Work out the finished part from the listing and answer in its coordinate system (mm). A direction names the side the tool comes from. Coordinates: 2 decimals unless noted, no trailing zeros. Order: outer loops, then holes, each group sorted by start corner. A loop starts at its lowest first (then second) coordinate and runs counter-clockwise, first axis right, second up.
```python
from build123d import *

# Parameters (mm, degrees)
F0_W      = 15
F0_H      = 15
F1_DEPTH  = 50
F2_W      = 15
F2_H      = 55
F3_DEPTH  = 20
F4_R      = 2.75
F5_DEPTH  = 50.001
F6_R      = 5
F7_DEPTH  = 45
F9_DEPTH  = 2.5
F10_R     = 1.5
F11_DEPTH = 12.501
F13_DEPTH = 2.5
F14_R     = 1.5
F15_DEPTH = 25
F16_R     = 5


with BuildPart() as f1:
    # F0 (on Front) → F1 (new body)
    with BuildSketch(Plane.XZ):
        with Locations((0, 20)):
            Rectangle(F0_W, F0_H)
        with Locations((0, -20)):
            Rectangle(F0_W, F0_H)
    extrude(amount=F1_DEPTH)

    # F2 (on face) → F3 (join)
    with BuildSketch(Plane.XZ.offset(50)):
        Rectangle(F2_W, F2_H)
    extrude(amount=-F3_DEPTH)

    # F4 (on face) → F5 (cut, through all)
    with BuildSketch(Plane(origin=(0, 0, 0), x_dir=(-1, 0, 0), z_dir=(0, 1, 0))):
        with Locations((0, 20)):
            Circle(F4_R)
        with Locations((0, -20)):
            Circle(F4_R)
    extrude(amount=-F5_DEPTH, mode=Mode.SUBTRACT)

    # F6 (on face) → F7 (cut)
    with BuildSketch(Plane.XZ.offset(50)):
        with Locations((0, 20)):
            Circle(F6_R)
        with Locations((0, -20)):
            Circle(F6_R)
    extrude(amount=-F7_DEPTH, mode=Mode.SUBTRACT)

    # F8 (on face) → F9 (cut)
    with BuildSketch(Plane(origin=(-7.5, 0, 0), x_dir=(0, -1, 0), z_dir=(-1, 0, 0))):
        Polygon((35.5, -3.175426), (38.25, -1.587713), (38.25, 1.587713), (35.5, 3.175426), (32.75, 1.587713), (32.75, -1.587713), align=None)
        Polygon((47.25, 1.587713), (44.5, 3.175426), (41.75, 1.587713), (41.75, -1.587713), (44.5, -3.175426), (47.25, -1.587713), align=None)
    extrude(amount=-F9_DEPTH, mode=Mode.SUBTRACT)

    # F10 (on face) → F11 (cut, through all)
    with BuildSketch(Plane(origin=(-5, 0, 0), x_dir=(0, -1, 0), z_dir=(-1, 0, 0))):
        with Locations((35.5, 0)):
            Circle(F10_R)
        with Locations((44.5, 0)):
            Circle(F10_R)
    extrude(amount=-F11_DEPTH, mode=Mode.SUBTRACT)

    # F12 (on face) → F13 (cut)
    with BuildSketch(Plane.XZ.offset(50)):
        Polygon((1.587713, 2), (3.175426, 4.75), (1.587713, 7.5), (-1.587713, 7.5), (-3.175426, 4.75), (-1.587713, 2), align=None)
        Polygon((1.587713, -7.5), (3.175426, -4.75), (1.587713, -2), (-1.587713, -2), (-3.175426, -4.75), (-1.587713, -7.5), align=None)
    extrude(amount=-F13_DEPTH, mode=Mode.SUBTRACT)

    # F14 (on face) → F15 (cut)
    with BuildSketch(Plane.XZ.offset(47.5)):
        with Locations((0, 4.75)):
            Circle(F14_R)
        with Locations((0, -4.75)):
            Circle(F14_R)
    extrude(amount=-F15_DEPTH, mode=Mode.SUBTRACT)

    # F16
    f16_edges = [f1.edges().sort_by_distance(p)[0] for p in [
        (0, -30, 12.5),
        (0, -30, -12.5),
    ]]
    fillet(f16_edges, radius=F16_R)


solid = f1.part
```
1. Flat-ended cylindrical pins translate along their axes: pin 1 (3.5 mm diameter, centred on x = 0, z = -20, fed in from +Y); pin 2 (6 mm diameter, centred on x = 0.5, z = 5.5, fed in from -Y); pin 3 (3.5 mm diameter, centred on x = 0, z = -4.75, fed in from +Y); pin 4 (9 mm diameter, centred on x = 0, z = 20, fed in from -Y). Find the tip coordinate at first contact, or state that the pin passes through.
2. The part is cut by section A-A (y = -21). Determine the outline of the cut face in (x, z), plus the area to 3 significant figures.
3. The part is cut by section C-C (z = 20). Determine the outline of the cut face in (x, y).
4. Consider probe 1 along Z at (x, y) = (0.25, -8); probe 2 along Z at (x, y) = (0, -1.25); probe 3 along Z at (x, y) = (0, -37.5). Determine where each line is inside the solid, lowest interval first.
5. The part is cut by section D-D (y = -39.5). Determine the outline of the cut face in (x, z).
6. The part is cut by section B-B (z = 0). Determine the outline of the cut face in (x, y), plus the area to 4 significant figures.
7. The mould has two halves that part along Z. Classify faces 1 (the flat face through (0, -25, -27.5)), 2 (the flat face through (0, -49, 7.5)): released by +Z, released by -Z, zero draft, split by the parting line, or undercut.
8. For faces 3 (the flat face through (2.2, -5, 17.8)), 4 (the cylindrical face through (-1.5, -38.9, 4.8)), 5 (the flat face through (-6.268, -45.894, 2.37)), determine the directions among +Z, -Z, +X, -X, +Y, -Y from which every point of the face is accessible in a straight line to the end or side of a thin tool.
Worked out:
1. pin 1: passes through
1. pin 2: stops at y = -50
1. pin 3: stops at y = -30
1. pin 4: stops at y = -5
2. outline: (-7.5, -27.5) - (7.5, -27.5) - (7.5, -12.5) - (-7.5, -12.5) - close; (-7.5, 12.5) - (7.5, 12.5) - (7.5, 27.5) - (-7.5, 27.5) - close; hole circle Ø10 at (0, -20); hole circle Ø10 at (0, 20)
2. area: 293 mm2
3. outline: (-7.5, -50) - (-5, -50) - (-5, -5) - (-2.75, -5) - (-2.75, 0) - (-7.5, 0) - close; (2.75, -5) - (5, -5) - (5, -50) - (7.5, -50) - (7.5, 0) - (2.75, 0) - close
4. probe 1: z = -27.5 to -24.99, -15.01 to -12.5, 12.5 to 15.01, 24.99 to 27.5
4. probe 2: z = -27.5 to -22.75, -17.25 to -12.5, 12.5 to 17.25, 22.75 to 27.5
4. probe 3: z = -27.5 to -25, -15 to -6.25, -3.25 to 3.25, 6.25 to 15, 25 to 27.5
5. outline: (-7.5, -27.5) - (7.5, -27.5) - (7.5, 27.5) - (-7.5, 27.5) - close; hole circle Ø10 at (0, -20); hole circle Ø10 at (0, 20); hole circle Ø3 at (0, -4.75); hole circle Ø3 at (0, 4.75)
6. outline: (-7.5, -50) - (7.5, -50) - (7.5, -46) - (-5, -46) - (-5, -47.25) - (-7.5, -47.25) - close; (-7.5, -41.75) - (-5, -41.75) - (-5, -43) - (7.5, -43) - (7.5, -37) - (-5, -37) - (-5, -38.25) - (-7.5, -38.25) - close; (-7.5, -32.75) - (-5, -32.75) - (-5, -34) - (7.5, -34) - (7.5, -30) - (-7.5, -30) - close
6. area: 197.5 mm2
7. face 1: released by -Z
7. face 2: undercut
8. face 3: -Y
8. face 4: +Y, -Y
8. face 5: -X
